Source: CAD feature listing. Evaluate the final solid. Frame: model axes, mm. A direction names the side the tool comes from. Give positions to 0.01 mm unless a question says otherwise; leave off trailing zeros. Write each loop counter-clockwise with the first axis right and the second up, starting at its lowest first coordinate (ties: lowest second). Pieces come first, ordered by that corner, then holes. Notation, with made-up numbers: (-20, 85) -> (37, 85) arc R24 cw to (37, 113) -> close; hole circle Ø9 at (-37, 83.5). An arc over 180 degrees is marked (long way). Write item = value, one per line.
from build123d import *

# Parameters (mm, degrees)
F0_W      = 64
F0_H      = 87
F1_DEPTH  = 13
F3_DEPTH  = 7
F5_DEPTH  = 29.5
F7_DEPTH  = 29.5
F9_DEPTH  = 5
F10_DEPTH = 5
F12_DEPTH = 64.001


with BuildPart() as f1:
    # F0 (on Front) → F1 (new body)
    with BuildSketch(Plane.XZ):
        with Locations((1.2601554287, 25.9569030584)):
            Rectangle(F0_W, F0_H)
    extrude(amount=-F1_DEPTH)

    # F2 (on face) → F3 (cut)
    with BuildSketch(Plane(origin=(0, 13, 0), x_dir=(-1, 0, 0), z_dir=(0, 1, 0))):
        Polygon((-11.2601554287, 33.9569030584), (-33.2601554287, 33.9569030584), (-33.2601554287, 31.7069030584), (-32.2601554287, 32.4569030584), (-31.2601554287, 31.7069030584), (-30.2601554287, 32.4569030584), (-29.2601554287, 31.7069030584), (-28.2601554287, 32.4569030584), (-27.2601554287, 31.7069030584), (-26.2601554287, 32.4569030584), (-25.2601554287, 31.7069030584), (-24.2601554287, 32.4569030584), (-23.2601554287, 31.7069030584), (-22.2601554287, 32.4569030584), (-21.2601554287, 31.7069030584), (-20.2601554287, 32.4569030584), (-19.2601554287, 31.7069030584), (-18.2601554287, 32.4569030584), (-17.2601554287, 31.7069030584), (-16.2601554287, 32.4569030584), (-15.2601554287, 31.7069030584), (-14.2601554287, 32.4569030584), (-13.2601554287, 31.7069030584), (-12.2601554287, 32.4569030584), (-11.2601554287, 31.7069030584), align=None)
        Polygon((8.7398445713, 33.9569030584), (-11.2601554287, 33.9569030584), (-11.2601554287, 31.7069030584), (-10.2601554287, 32.4569030584), (-9.2601554287, 31.7069030584), (-8.2601554287, 32.4569030584), (-7.2601554287, 31.7069030584), (-6.2601554287, 32.4569030584), (-5.2601554287, 31.7069030584), (-4.2601554287, 32.4569030584), (-3.2601554287, 31.7069030584), (-2.2601554287, 32.4569030584), (-1.2601554287, 31.7069030584), (-0.2601554287, 32.4569030584), (0.7398445713, 31.7069030584), (1.7398445713, 32.4569030584), (2.7398445713, 31.7069030584), (3.7398445713, 32.4569030584), (4.7398445713, 31.7069030584), (5.7398445713, 32.4569030584), (6.7398445713, 31.7069030584), (7.7398445713, 32.4569030584), (8.7398445713, 31.7069030584), align=None)
        Polygon((-9.2601554287, 31.7069030584), (-11.2601554287, 31.7069030584), (-11.2601554287, 25.9569030584), (8.7398445713, 25.9569030584), (8.7398445713, 31.7069030584), (6.7398445713, 31.7069030584), (4.7398445713, 31.7069030584), (2.7398445713, 31.7069030584), (0.7398445713, 31.7069030584), (-1.2601554287, 31.7069030584), (-3.2601554287, 31.7069030584), (-5.2601554287, 31.7069030584), (-7.2601554287, 31.7069030584), align=None)
        Polygon((30.7398445713, 33.9569030584), (8.7398445713, 33.9569030584), (8.7398445713, 31.7069030584), (9.7398445713, 32.4569030584), (10.7398445713, 31.7069030584), (11.7398445713, 32.4569030584), (12.7398445713, 31.7069030584), (13.7398445713, 32.4569030584), (14.7398445713, 31.7069030584), (15.7398445713, 32.4569030584), (16.7398445713, 31.7069030584), (17.7398445713, 32.4569030584), (18.7398445713, 31.7069030584), (19.7398445713, 32.4569030584), (20.7398445713, 31.7069030584), (21.7398445713, 32.4569030584), (22.7398445713, 31.7069030584), (23.7398445713, 32.4569030584), (24.7398445713, 31.7069030584), (25.7398445713, 32.4569030584), (26.7398445713, 31.7069030584), (27.7398445713, 32.4569030584), (28.7398445713, 31.7069030584), (29.7398445713, 32.4569030584), (30.7398445713, 31.7069030584), align=None)
        Polygon((-11.2601554287, 25.9569030584), (-33.2601554287, 25.9569030584), (-33.2601554287, 19.9569030584), (30.7398445713, 19.9569030584), (30.7398445713, 25.9569030584), (8.7398445713, 25.9569030584), align=None)
        Polygon((6.7398445713, 31.7069030584), (8.7398445713, 31.7069030584), (7.7398445713, 32.4569030584), align=None)
        Polygon((4.7398445713, 31.7069030584), (6.7398445713, 31.7069030584), (5.7398445713, 32.4569030584), align=None)
        Polygon((2.7398445713, 31.7069030584), (4.7398445713, 31.7069030584), (3.7398445713, 32.4569030584), align=None)
        Polygon((0.7398445713, 31.7069030584), (2.7398445713, 31.7069030584), (1.7398445713, 32.4569030584), align=None)
        Polygon((-1.2601554287, 31.7069030584), (0.7398445713, 31.7069030584), (-0.2601554287, 32.4569030584), align=None)
        Polygon((-2.2601554287, 32.4569030584), (-3.2601554287, 31.7069030584), (-1.2601554287, 31.7069030584), align=None)
        Polygon((-6.2601554287, 32.4569030584), (-7.2601554287, 31.7069030584), (-5.2601554287, 31.7069030584), align=None)
        Polygon((-4.2601554287, 32.4569030584), (-5.2601554287, 31.7069030584), (-3.2601554287, 31.7069030584), align=None)
        Polygon((-8.2601554287, 32.4569030584), (-9.2601554287, 31.7069030584), (-7.2601554287, 31.7069030584), align=None)
        Polygon((-10.2601554287, 32.4569030584), (-11.2601554287, 31.7069030584), (-9.2601554287, 31.7069030584), align=None)
    extrude(amount=-F3_DEPTH, mode=Mode.SUBTRACT)

    # F4 (on face) → F5 (cut, through all)
    with BuildSketch(Plane(origin=(-30.7398445713, 0, 0), x_dir=(0, -1, 0), z_dir=(-1, 0, 0))):
        with BuildLine():
            ThreePointArc((-13, 44.4569030584), (-7.6966991411, 46.6536021995), (-5.5, 51.9569030584))
            ThreePointArc((-5.5, 51.9569030584), (-7.6966991411, 57.2602039173), (-13, 59.4569030584))
            Line((-13, 59.4569030584), (-13, 44.4569030584))
        make_face()
    extrude(amount=-F5_DEPTH, mode=Mode.SUBTRACT)

    # F6 (on face) → F7 (cut, through all)
    with BuildSketch(Plane.YZ.offset(33.2601554287)):
        with BuildLine():
            Line((13, 44.2069030584), (13, 59.2069030584))
            ThreePointArc((13, 59.2069030584), (5.5, 51.7069030584), (13, 44.2069030584))
        make_face()
    extrude(amount=-F7_DEPTH, mode=Mode.SUBTRACT)

    # F8 (on face) → F9 (join)
    with BuildSketch(Plane.YZ.offset(33.2601554287)):
        with BuildLine():
            Line((13, 59.2069030584), (13, 64.3319030584))
            Line((13, 64.3319030584), (0, 64.3319030584))
            Line((0, 64.3319030584), (0, 38.0137264729))
            Line((0, 38.0137264729), (13, 38.0137264729))
            Line((13, 38.0137264729), (13, 44.2069030584))
            ThreePointArc((13, 44.2069030584), (5.5, 51.7069030584), (13, 59.2069030584))
        make_face()
        with BuildLine():
            Line((13, 44.2069030584), (13, 59.2069030584))
            ThreePointArc((13, 59.2069030584), (5.5, 51.7069030584), (13, 44.2069030584))
        make_face()
    extrude(amount=-F9_DEPTH)

    # F4 (on face) → F10 (join)
    with BuildSketch(Plane(origin=(-30.7398445713, 0, 0), x_dir=(0, -1, 0), z_dir=(-1, 0, 0))):
        with BuildLine():
            ThreePointArc((-13, 44.4569030584), (-7.6966991411, 46.6536021995), (-5.5, 51.9569030584))
            ThreePointArc((-5.5, 51.9569030584), (-7.6966991411, 57.2602039173), (-13, 59.4569030584))
            Line((-13, 59.4569030584), (-13, 44.4569030584))
        make_face()
    extrude(amount=-F10_DEPTH)

    # F11 (on face) → F12 (cut, through all)
    with BuildSketch(Plane(origin=(-30.7398445713, 0, 0), x_dir=(0, -1, 0), z_dir=(-1, 0, 0))):
        with BuildLine():
            ThreePointArc((-13, 46.9569030584), (-9.4644660941, 48.4213691524), (-8, 51.9569030584))
            ThreePointArc((-8, 51.9569030584), (-9.4644660941, 55.4924369643), (-13, 56.9569030584))
            Line((-13, 56.9569030584), (-13, 46.9569030584))
        make_face()
    extrude(amount=-F12_DEPTH, mode=Mode.SUBTRACT)


solid = f1.part
(1) Pull-direction query (X, two-part tool) for faces 4 (the face through (-30.74, 7, 27)), 5 (the face through (2, 6, 25)), 6 (the face through (1, 6, 69.457)), 7 (the face through (3.76, 7.5, 51.8)); classes: pulls with the +X half, pulls with the -X half, needs draft (parallel to the pull), parting line crosses it, or undercut.
Values follow:
face_4 = pulls with the -X half
face_5 = undercut
face_6 = needs draft
face_7 = undercut
(2) Material intervals for line 1 (Z direction, x = -5, y = 11.5); line 2 (Z direction, x = 24.5, y = 12.25); line 3 (Z direction, x = -18, y = 10.75), sorted ascending.
Values follow:
line_1 = -17.54 to 19.96, 33.96 to 44.61, 59.31 to 69.46
line_2 = -17.54 to 19.96, 25.96 to 32.28, 33.96 to 44.24, 59.17 to 69.46
line_3 = -17.54 to 19.96, 25.96 to 32.26, 33.96 to 44.8, 59.11 to 69.46
(3) Section query A-A (x = -5). Return loops of the section in (y, z), plus the area to 3 significant figures.
Values follow:
outline = (0, -17.54) -> (13, -17.54) -> (13, 19.96) -> (6, 19.96) -> (6, 33.96) -> (13, 33.96) -> (13, 44.46) arc R7.5 cw to (13, 59.46) -> (13, 69.46) -> (0, 69.46) -> close
area = 945 mm2
(4) Access query for faces 1 (the face through (2, 10, 19.957)), 2 (the face through (11.26, 10, 29)), 3 (the face through (1, 13, 65)). Directions: +Z, -Z, +X, -X, +Y, -Y. A direction counts if a zero-diameter tool reaches every point of the face in a straight line with its end or side. Return the directions, or none.
Values follow:
face_1 = +X, -X, +Y
face_2 = +Y
face_3 = +Z, -Z, +X, -X, +Y
(5) Section query B-B (y = 9.25). Give the number of separate pieces and of enclosed holes in the cut face, plus the area to 3 significant figures.
Values follow:
separate_pieces = 5
enclosed_holes = 0
area = 4,210 mm2
